Can you work these out from the model? Positions are in its coordinate system, mm. A direction names the side the tool comes from. Round coordinates to 2 decimals unless told otherwise and drop trailing zeros. Loops run counter-clockwise (first coordinate to the right, second up) from the corner with the lowest first, then second, coordinate; pieces in that order, holes last. Notation, with made-up numbers: M 30,-9 L 66,-9 A25 cw 66,24 Z; hole C 23.25,24 d9. An arc over 180 degrees is marked long. Use a Markdown table: item, result. Add a question column.
```python
from build123d import *

# Parameters (mm, degrees)
F0_R      = 1.1
F1_DEPTH  = 1.5
F3_DEPTH  = 1.5
F4_W      = 21.9317121995
F4_H      = 1.5
F5_DEPTH  = 5
F7_DEPTH  = 1.5
F9_DEPTH  = 1.5
F10_R     = 1
F11_W     = 27.487267755
F11_H     = 1.5
F12_DEPTH = 1.5
F14_DEPTH = 32
F17_R     = 1.1
F18_DEPTH = 1.5


with BuildPart() as f1:
    # F0 (on Top) → F1 (new body)
    with BuildSketch(Plane.XY):
        Polygon((11, 3.5), (11, 16.5), (-11, 16.5), (-11, 3.5), (-2, -16.5), (11, -16.5), align=None)
        with Locations((-8, 13.5)):
            Circle(F0_R, mode=Mode.SUBTRACT)
        with Locations((8, 13.5)):
            Circle(F0_R, mode=Mode.SUBTRACT)
        Polygon((20, -16.5), (11, 3.5), (11, -16.5), align=None)
    extrude(amount=F1_DEPTH)

    # F2 (on face) → F3 (cut, through all)
    with BuildSketch(Plane.XY.offset(1.5)):
        Polygon((13.0518233866, -1.0596075259), (3, -16.5), (20, -16.5), align=None)
        with BuildLine():
            Line((4, 10), (-4, 10))
            ThreePointArc((-4, 10), (-4.7071067812, 9.7071067812), (-5, 9))
            Line((-5, 9), (-5, 8))
            ThreePointArc((-5, 8), (-4.7071067812, 7.2928932188), (-4, 7))
            Line((-4, 7), (4, 7))
            ThreePointArc((4, 7), (4.7071067812, 7.2928932188), (5, 8))
            Line((5, 8), (5, 9))
            ThreePointArc((5, 9), (4.7071067812, 9.7071067812), (4, 10))
        make_face()
        with BuildLine():
            Line((4, 3), (-4, 3))
            ThreePointArc((-4, 3), (-4.7071067812, 2.7071067812), (-5, 2))
            Line((-5, 2), (-5, 1))
            ThreePointArc((-5, 1), (-4.7071067812, 0.2928932188), (-4, 0))
            Line((-4, 0), (4, 0))
            ThreePointArc((4, 0), (4.7071067812, 0.2928932188), (5, 1))
            Line((5, 1), (5, 2))
            ThreePointArc((5, 2), (4.7071067812, 2.7071067812), (4, 3))
        make_face()
        with BuildLine():
            Line((4, -4), (-4, -4))
            ThreePointArc((-4, -4), (-4.7071067812, -4.2928932188), (-5, -5))
            Line((-5, -5), (-5, -6))
            ThreePointArc((-5, -6), (-4.7071067812, -6.7071067812), (-4, -7))
            Line((-4, -7), (4, -7))
            ThreePointArc((4, -7), (4.7071067812, -6.7071067812), (5, -6))
            Line((5, -6), (5, -5))
            ThreePointArc((5, -5), (4.7071067812, -4.2928932188), (4, -4))
        make_face()
    extrude(amount=-F3_DEPTH, mode=Mode.SUBTRACT)

    # F4 (on face) → F5 (join)
    with BuildSketch(Plane(origin=(-7.8378378378, -3.527027027, 0), x_dir=(0.4103646773, -0.9119215052, 0), z_dir=(-0.9119215052, -0.4103646773, 0))):
        with Locations((3.260119381, 0.75)):
            Rectangle(F4_W, F4_H)
    extrude(amount=F5_DEPTH)

    # F6 (on face) → F7 (join)
    with BuildSketch(Plane.XY.offset(1.5)):
        Polygon((-2, -16.5), (-6.5596075259, -18.5518233866), (-4.2798037629, -23.618053971), (3, -23.618053971), (3, -16.5), align=None)
    extrude(amount=-F7_DEPTH)

    # F8 (on face) → F9 (cut, through all)
    with BuildSketch(Plane.XY.offset(1.5)):
        Polygon((3, -23.618053971), (3, -16.5), (-1.6339120908, -23.618053971), align=None)
    extrude(amount=-F9_DEPTH, mode=Mode.SUBTRACT)

    # F10
    f10_edges = [f1.edges().sort_by_distance(p)[0] for p in [
        (-11, 16.5, 0.75),
        (11, 16.5, 0.75),
        (-11, 3.5, 0.75),
        (-1.633912, -23.618054, 0.75),
        (13.051823, -1.059608, 0.75),
        (11, 3.5, 0.75),
    ]]
    fillet(f10_edges, radius=F10_R)

    # F11 (on face) → F12 (join)
    with BuildSketch(Plane(origin=(-12.3974453637, -5.5788504137, 0), x_dir=(0.4103646773, -0.9119215052, 0), z_dir=(-0.9119215052, -0.4103646773, 0))):
        with Locations((6.0378971588, 0.75)):
            Rectangle(F11_W, F11_H)
    extrude(amount=F12_DEPTH)

    # F13 (on face) → F14 (join)
    with BuildSketch(Plane(origin=(0, 0, 0), x_dir=(1, 0, 0), z_dir=(0, 0, -1))):
        Polygon((-15.5596075259, -1.4481766134), (-4.2798037629, 23.618053971), (-5.6476860207, 24.2336009869), (-16.9274897836, -0.8326295974), align=None)
    extrude(amount=F14_DEPTH)

    # F16: F1 across plane


with BuildPart() as f1_1:
    add(f1.part)
    add(f1.part.mirror(Plane.XY.offset(-15.25)))

    # F17 (on face) → F18 (cut, through all)
    with BuildSketch(Plane(origin=(-13.7653276215, -6.1943974297, 0), x_dir=(0.4103646773, -0.9119215052, 0), z_dir=(-0.9119215052, -0.4103646773, 0))):
        with Locations((-3.9621028412, -25.25)):
            Circle(F17_R)
        with Locations((16.0378971588, -25.25)):
            Circle(F17_R)
        with Locations((-3.9621028412, -5.25)):
            Circle(F17_R)
        with Locations((16.0378971588, -5.25)):
            Circle(F17_R)
    extrude(amount=-F18_DEPTH, mode=Mode.SUBTRACT)


solid = f1_1.part
```
(1) Thinking about a two-plate mould opening in Z: for faces 1 (the face through (-4.715, -6.699, 0.76)), 2 (the face through (-1, -1, -30.5)), which applies, released by +Z, released by -Z, zero draft, split by the parting line, or undercut?
(2) On a 3-axis mill with a long thin cutter (end or side, diameter ignored), from which of +Z, -Z, +X, -X, +Y, -Y can I reach the whole of each face in a straight line? I mean faces 3 (the face through (-14.815, -2.06, -26.324)), 4 (the face through (-10, -10.91, -15.04)), 5 (the face through (-5, 1.5, 0.8)). Say none if no direction works.
(3) Suppose I cut it at B-B on x = 1. Count the separate pieces of the cut face and the enclosed holes in it, and give its area (3 significant figures).
(4) I'm going to push flat-ended pins straight in: pin 1 (5 mm diameter, centred on x = -11, z = -9, fed in from -Y); pin 2 (10 mm diameter, centred on x = -2.5, z = -7, fed in from +Y); pin 3 (1.2 mm diameter, centred on x = -0.5, z = 1, fed in from -Y). Where does each tip first touch, or does it pass through?
(5) If I drill on probe 1 along Z at (x, y) = (-1.5, -22); probe 2 along X at (y, z) = (8, -31); probe 3 along Y at (x, z) = (-8, -31.4), over which ranges is the centre line in solid material (lowest first)? Write a range as [from, to].
(6) Suppose I cut it at D-D on x = 8. List the corners of the cut face in (y, z) for me, and give its area (3 significant figures).
(7) Suppose I cut it at C-C on y = 6.5. List the corners of the cut face in (x, z) for me, and give its area (3 significant figures).
(8) Suppose I cut it at A-A on y = 13.5. List the corners of the cut face in (x, z) for me.
Results below:
| question | item | result |
|---|---|---|
| 1 | face 1 | zero draft |
| 1 | face 2 | undercut |
| 2 | face 3 | none |
| 2 | face 4 | +X, +Y |
| 2 | face 5 | +Z, -Z |
| 3 | separate pieces | 8 |
| 3 | enclosed holes | 0 |
| 3 | area | 81.2 mm² |
| 4 | pin 1 | stops at y = -17.9 |
| 4 | pin 2 | stops at y = -16.46 |
| 4 | pin 3 | stops at y = -22.8 |
| 5 | probe 1 | z = [-32, -30.5], [0, 1.5] |
| 5 | probe 2 | x = [-11, -5], [5, 11] |
| 5 | probe 3 | y = [-19.01, 12.4], [14.6, 16.5] |
| 6 | outline | M -8.82,-32 L 12.4,-32 L 12.4,-30.5 L -8.82,-30.5 Z; M -8.82,0 L 12.4,0 L 12.4,1.5 L -8.82,1.5 Z; M 14.6,-32 L 16.5,-32 L 16.5,-30.5 L 14.6,-30.5 Z; M 14.6,0 L 16.5,0 L 16.5,1.5 L 14.6,1.5 Z |
| 6 | area | 69.4 mm² |
| 7 | outline | M -11,-32 L 11,-32 L 11,-30.5 L -11,-30.5 Z; M -11,0 L 11,0 L 11,1.5 L -11,1.5 Z |
| 7 | area | 66.0 mm² |
| 8 | outline | M -11,-32 L -9.1,-32 L -9.1,-30.5 L -11,-30.5 Z; M -11,0 L -9.1,0 L -9.1,1.5 L -11,1.5 Z; M -6.9,-32 L 6.9,-32 L 6.9,-30.5 L -6.9,-30.5 Z; M -6.9,0 L 6.9,0 L 6.9,1.5 L -6.9,1.5 Z; M 9.1,-32 L 11,-32 L 11,-30.5 L 9.1,-30.5 Z; M 9.1,0 L 11,0 L 11,1.5 L 9.1,1.5 Z |
